```python
from build123d import *

# Parameters (mm, degrees)
SKETCH18_R                      = 11.825
EXTRUDE17_DEPTH                 = 1.6129
SKETCH19_R                      = 3.4
EXTRUDE19_DEPTH                 = 4.1
SKETCH20_R                      = 0.5
SKETCH20_R_2                    = 1.27
EXTRUDE20_DEPTH                 = 5.1
SKETCH23_R                      = 0.5
CUT_EXTRUDE1_DEPTH              = 5.1
CIRPATTERN1_COUNT               = 2
CIRPATTERN1_ANGLE               = 22.5
CIRPATTERN1_THE_OTHER_WAY_COUNT = 2
CIRPATTERN1_THE_OTHER_WAY_ANGLE = 22.5
MIRROR2_COPY_1_SKETCH_R         = 0.5
MIRROR2_COPY_1_DEPTH            = 5.1
MIRROR2_COPY_2_SKETCH_R         = 0.5
MIRROR2_COPY_2_DEPTH            = 5.1
SKETCH21_R                      = 2.44475
EXTRUDE21_DEPTH                 = 1.1557
SKETCH22_R                      = 2.286
EXTRUDE22_DEPTH                 = 2.3368
EXTRUDE22_TAPER                 = 5
SKETCH24_R                      = 2.69475
SKETCH24_R_2                    = 2.44475
BOSS_EXTRUDE1_DEPTH             = 0.25
FILLET1_R                       = 0.5


with BuildPart() as part:
    # Sketch18 → Extrude17 (new body)
    with BuildSketch(Plane(origin=(0, 0, 0), x_dir=(1, 0, 0), z_dir=(0, 1, 0))):
        Circle(SKETCH18_R)
    extrude(amount=EXTRUDE17_DEPTH)

    # Sketch19 → Extrude19 (add)
    with BuildSketch(Plane(origin=(0, 1.6129, 0), x_dir=(1, 0, 0), z_dir=(0, 1, 0))):
        Circle(SKETCH19_R)
    extrude(amount=-EXTRUDE19_DEPTH)

    # Sketch20 → Extrude20 (cut, through all)
    with BuildSketch(Plane(origin=(0, 1.6129, 0), x_dir=(1, 0, 0), z_dir=(0, 1, 0))):
        with Locations((-9, 0)):
            Circle(SKETCH20_R)
        Circle(SKETCH20_R_2)
        with Locations((-8.314915793, 3.444150891)):
            Circle(SKETCH20_R)
        with Locations((-8.314915793, -3.444150891)):
            Circle(SKETCH20_R)
    extrude20 = extrude(amount=-EXTRUDE20_DEPTH, mode=Mode.SUBTRACT)

    # Mirror1: Extrude20 across plane
    add(extrude20.mirror(Plane(origin=(0, 0, 0), x_dir=(0, 0, 1), z_dir=(1, 0, 0))), mode=Mode.SUBTRACT)

    # Sketch23 → Cut-Extrude1 (cut, through all)
    with BuildSketch(Plane(origin=(0, 1.6129, 0), x_dir=(1, 0, 0), z_dir=(0, 1, 0))):
        with Locations((0, 8.2)):
            Circle(SKETCH23_R)
        with Locations((0, 10)):
            Circle(SKETCH23_R)
    cut_extrude1 = extrude(amount=-CUT_EXTRUDE1_DEPTH, mode=Mode.SUBTRACT)

    # CirPattern1: Cut-Extrude1 ×2 about axis
    cirpattern1_axis = Axis((0, 0, 0), (0, 1, 0))
    for i in range(1, CIRPATTERN1_COUNT):
        add(cut_extrude1.rotate(cirpattern1_axis, i * CIRPATTERN1_ANGLE / (CIRPATTERN1_COUNT - 1)), mode=Mode.SUBTRACT)

    # CirPattern1 the other way: Cut-Extrude1 ×2 about axis
    cirpattern1_the_other_way_axis = Axis((0, 0, 0), (0, -1, 0))
    for i in range(1, CIRPATTERN1_THE_OTHER_WAY_COUNT):
        add(cut_extrude1.rotate(cirpattern1_the_other_way_axis, i * CIRPATTERN1_THE_OTHER_WAY_ANGLE / (CIRPATTERN1_THE_OTHER_WAY_COUNT - 1)), mode=Mode.SUBTRACT)

    # Mirror2: Cut-Extrude1 across plane
    add(cut_extrude1.mirror(Plane.XY), mode=Mode.SUBTRACT)

    # Mirror2 copy 1 sketch → Mirror2 copy 1 (cut, through all)
    with BuildSketch(Plane(origin=(0, 1.6129, 0), x_dir=(0.923879533, 0, 0.382683432), z_dir=(0, 1, 0))):
        with Locations((0, -8.2)):
            Circle(MIRROR2_COPY_1_SKETCH_R)
        with Locations((0, -10)):
            Circle(MIRROR2_COPY_1_SKETCH_R)
    extrude(amount=-MIRROR2_COPY_1_DEPTH, mode=Mode.SUBTRACT)

    # Mirror2 copy 2 sketch → Mirror2 copy 2 (cut, through all)
    with BuildSketch(Plane(origin=(0, 1.6129, 0), x_dir=(0.923879533, 0, -0.382683432), z_dir=(0, 1, 0))):
        with Locations((0, -8.2)):
            Circle(MIRROR2_COPY_2_SKETCH_R)
        with Locations((0, -10)):
            Circle(MIRROR2_COPY_2_SKETCH_R)
    extrude(amount=-MIRROR2_COPY_2_DEPTH, mode=Mode.SUBTRACT)

    # Sketch21 → Extrude21 (cut)
    with BuildSketch(Plane(origin=(0, 1.6129, 0), x_dir=(1, 0, 0), z_dir=(0, 1, 0))):
        Circle(SKETCH21_R)
    extrude(amount=-EXTRUDE21_DEPTH, mode=Mode.SUBTRACT)

    # Sketch22 → Extrude22 (cut)
    with BuildSketch(Plane.XZ.offset(2.4871)):
        Circle(SKETCH22_R)
    extrude(amount=-EXTRUDE22_DEPTH, taper=EXTRUDE22_TAPER, mode=Mode.SUBTRACT)

    # Sketch24 → Boss-Extrude1 (add)
    with BuildSketch(Plane(origin=(0, 1.6129, 0), x_dir=(1, 0, 0), z_dir=(0, 1, 0))):
        Circle(SKETCH24_R)
        Circle(SKETCH24_R_2, mode=Mode.SUBTRACT)
    extrude(amount=BOSS_EXTRUDE1_DEPTH)

    # Fillet1
    fillet1_edges = [part.edges().sort_by_distance(p)[0] for p in [
        (-3.4, 0, 0),
    ]]
    fillet(fillet1_edges, radius=FILLET1_R)


solid = part.part
```
Here's how the part is built. I have some questions about the finished solid (model axes, mm). A direction names the side the tool comes from. Round coordinates to 2 decimals unless told otherwise and drop trailing zeros. Write each loop counter-clockwise with the first axis right and the second up, starting at its lowest first coordinate (ties: lowest second). Pieces come first, ordered by that corner, then holes. Notation, with made-up numbers: M 33,-37 L 63,-37 A30 ccw 63,2 Z; hole C -30,53.5 d11. An arc over 180 degrees is marked long. Answer as CSV lines item,"result". Start each with the question number.
1. Suppose I cut it at A-A on z = 0. Count the separate pieces of the cut face and the enclosed holes in it, then the cut area to 3 significant figures.
2. On a 3-axis mill with a long thin cutter (end or side, diameter ignored), from which of +Z, -Z, +X, -X, +Y, -Y can I reach the whole of each face in a straight line? I mean faces 1 (the cylindrical face through (-8.423, 0.818, -2.956)), 2 (the cylindrical face through (-0.53, 1.15, 2.387)). Say none if no direction works.
3. I'm going to push flat-ended pins straight in: pin 1 Ø2 at (x, z) = (0.5, -0.5) entering from -Y; pin 2 Ø1.5 at (x, z) = (-8, -1) entering from +Y; pin 3 Ø1.5 at (x, y) = (4.5, 0.5) entering from +Z. Where does each tip first touch, or does it pass through?
4. Suppose I cut it at C-C on y = -1.3. Write out the boundary of the cut face in (x, z).
5. I need wall thicknesses on probe 1 along Z at (x, y) = (0, 1.2) (3 decimals); probe 2 along X at (y, z) = (0.9, 0) (3 decimals); probe 3 along Z at (x, y) = (8.25, 1.15). Which ranges of each line are inside material? Lowest first, please.
6. Thinking about a two-plate mould opening in Z: for faces 3 (the cylindrical face through (-0.108, 0.818, 9.512)), 4 (the cylindrical face through (-2.563, 0.795, 11.544)), which applies, released by +Z, released by -Z, zero draft, split by the parting line, or undercut?
7. Suppose I cut it at D-D on x = 7. Write out the boundary of the cut face in (y, z).
Check result:
1,separate pieces,"4"
1,enclosed holes,"0"
1,area,"34.7 mm2"
2,face 1,"+Y, -Y"
2,face 2,"+Y"
3,pin 1,"stops at y = -0.15"
3,pin 2,"stops at y = 1.61"
3,pin 3,"stops at z = 11.21"
4,outline,"C 0,0 d6.8; hole C 0,0 d4.36"
5,probe 1,"z = -11.825 to -10.5, -9.5 to -8.7, -7.7 to -2.445, 2.445 to 7.7, 8.7 to 9.5, 10.5 to 11.825"
5,probe 2,"x = -11.825 to -9.5, -8.5 to -2.445, 2.445 to 8.5, 9.5 to 11.825"
5,probe 3,"z = -8.47 to -3.94, -2.95 to 2.95, 3.94 to 8.47"
6,face 3,"undercut"
6,face 4,"split by the parting line"
7,outline,"M 0,-9.53 L 1.61,-9.53 L 1.61,9.53 L 0,9.53 Z"
